Build history of the part. All positions in model axes, mm. Round coordinates to 2 decimals unless told otherwise and drop trailing zeros. Order: outer loops, then holes, each group sorted by start corner. A loop starts at its lowest first (then second) coordinate and runs counter-clockwise, first axis right, second up. Notation, with made-up numbers: M 61.5,38.25 L 70.5,38.25 A23 cw 70.5,63.25 Z; hole C 39.5,87 d3. An arc over 180 degrees is marked long. One line per item, written item: value. Start each with the question number.
Item 1: Band-saw the part on A-A, the plane y = 0. Write the cut outline in (x, z), then the cut area to 3 significant figures.
Item 2: Band-saw the part on B-B, the plane z = 502.5. Write the cut outline in (x, y), then the cut area to 3 significant figures.
Item 3: Probe L1, parallel to X at y = -14.55, z = 601; L2, parallel to Y at x = 11.5, z = 1137. List the from-to ranges inside material, lowest first.
Item 4: Pin check, flat tips, straight feed: pin 1 (6 mm diameter, centred on x = 0, z = 1187, fed in from -Y); pin 2 (4 mm diameter, centred on x = 9.5, y = 9.5, fed in from -Z). Stop position of each tip, or through.
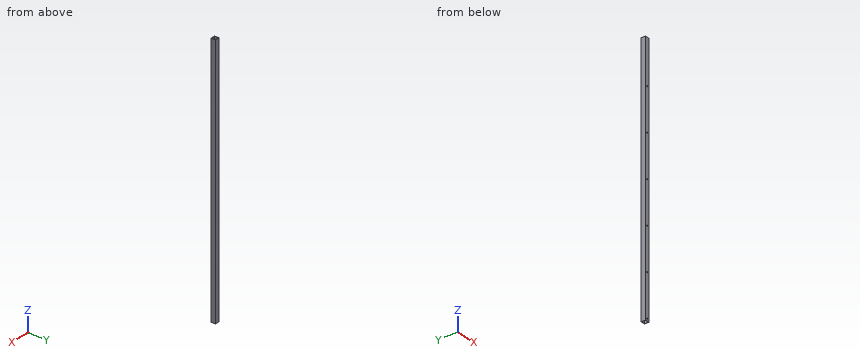
Autodesk Inventor part; units mm, degrees
ref_plane "YZ Plane" through (0, 0, 0) normal (1, 0, 0) x (0, 1, 0)
ref_plane "XZ Plane" through (0, 0, 0) normal (0, 1, 0) x (-1, 0, 0)
ref_plane "XY Plane" through (0, 0, 0) normal (0, 0, 1) x (1, 0, 0)
sketch "Náčrt1" plane through (0, 0, 0) normal (0, 0, 1) x (1, 0, 0)
  line L0 (-15, -15) -> (15, -15)
  line L1 (15, -15) -> (15, 15)
  line L2 (15, 15) -> (-15, 15)
  line L3 (-15, 15) -> (-15, -15)
  line L4 (-15, -15) -> (15, 15) construction
  line L5 (15, -15) -> (-15, 15) construction
  line L6 (-13, -13) -> (13, -13)
  line L7 (13, -13) -> (13, 13)
  line L8 (13, 13) -> (-13, 13)
  line L9 (-13, 13) -> (-13, -13)
  line L10 (-13, -13) -> (13, 13) construction
  line L11 (13, -13) -> (-13, 13) construction
  point P0 (0, 0)
  dimension "d0" = 30
  dimension "d1" = 30
  dimension "d2" = 26
  dimension "d3" = 26
extrude "Vysunutí1" add sketch "Náčrt1" along normal blind 1790
sketch "Náčrt2" plane through (-15, 15, 0) normal (0, 1, 0) x (1, 0, 0)
  circle A0 centre (15, -15) radius 1.5
  line L0 (30, 0) -> (0, 0)
  line L1 (0, 0) -> (0, -1790)
  line L2 (30, -1790) -> (0, -1790)
  line L3 (30, 0) -> (30, -1790)
  point P0 (15, 0)
  dimension "d8" = 3
  dimension "d13" = 15
  dimension "d19" = 15
extrude "Vysunutí2" cut sketch "Náčrt2" against normal up to surface (2 mm away) contours A0
sketch "Náčrt3" plane through (-15, -15, 0) normal (0, -1, 0) x (1, 0, 0)
  line L0 (30, 0) -> (0, 0)
  line L1 (0, 0) -> (0, 1790)
  line L2 (30, 1790) -> (0, 1790)
  line L3 (30, 0) -> (30, 1790)
  circle A0 centre (15, 15) radius 1.5
  circle A1 centre (15, 15) radius 5
  point P0 (15, 0)
  dimension "d15" = 10
extrude "Vysunutí3" cut sketch "Náčrt3" against normal up to surface (2 mm away) contours A0 | A1
pattern_linear "Obdélníkové pole1" count 6 spacing 293 along (0, 0, 1) of "Vysunutí2"
pattern_linear "Obdélníkové pole3" count 6 spacing 293 along (0, 0, 1) of "Vysunutí3"
equation "\"d0\" = width"
equation "\"d1\" = width"
equation "\"d2\" = width - 2 * thickness"
equation "\"d3\" = width - 2 * thickness"
equation "\"d4\" = length"
equation "\"d8\" = holeDia"
equation "\"d13\" = holeOffset"
equation "\"d19\" = 0.5 * width"
equation "\"d15\" = holeDiaOpposite"
equation "\"d22\" = holeDistance"
equation "\"d28\" = holeDistance"
equation "\"width\" = gSquareProfile_Width_Rack"
equation "\"thickness\" = gSquareProfile_Thickness_Rack"
equation "\"length\" = gRack_Rom_Height - 2 * width"
equation "\"holeDistance\" = 293"
equation "\"holeDiaOpposite\" = 10"
equation "\"holeDia\" = 3"
equation "\"holeOffset\" = 0.5 * width"
properties part number "Profile-Square#16"
Output:
1. outline: M -15,0 L -13,0 L -13,1790 L -15,1790 Z; M 13,0 L 15,0 L 15,1790 L 13,1790 Z
1. area: 7,160 mm²
2. outline: M -15,-15 L 15,-15 L 15,15 L -15,15 Z; hole M -13,-13 L 13,-13 L 13,13 L -13,13 Z
2. area: 224 mm²
3. L1: x = -15 to -5, 5 to 15
3. L2: y = -15 to -13, 13 to 15
4. pin 1: stops at y = 13
4. pin 2: passes through
